The model under review builds one solid part; all positions refer to its coordinate system, in mm. A direction names the side the tool comes from. Give positions to 0.01 mm unless a question says otherwise; leave off trailing zeros. Order: outer loops, then holes, each group sorted by start corner. A loop starts at its lowest first (then second) coordinate and runs counter-clockwise, first axis right, second up. Notation, with made-up numbers: (56, 66.25) - (102, 66.25) arc R20 ccw to (102, 70.25) - close; hole circle Ø2 at (40.5, -0.75). An arc over 180 degrees is marked (long way). Write item = value, one per line. Start each with the question number.
1. For P1, Ø5, axis at y = 38, z = 5.5, coming from the +X side; P2, Ø4.5, axis at x = 55.5, z = 10, coming from the +Y side, all flat-tipped, find the tip position at first contact; note any pin that passes through.
2. Machinability: for faces 1 (the cylindrical face through (126.82, 51.02, 7.4)), 2 (the flat face through (43, 50, 7)), which of the approach directions +Z, -Z, +X, -X, +Y, -Y give a long, thin tool a straight path to every point of the face, cutting with its end or side? Answer none if there is none.
3. We need section A-A, the plane z = 7.5. Give the boundary of the cut face in (x, y).
4. We need section B-B, the plane x = 61.5. Give the boundary of the cut face in (y, z), and give its area (3 significant figures).
5. Wall thickness on probe 1 along Y at (x, z) = (40.5, 5.5); probe 2 along Y at (x, z) = (5.5, 8.5); probe 3 along X at (y, z) = (22.5, 10.5): over which ranges is each line inside the solid? List them lowest first.
6. We need section C-C, the plane y = 17.5. Give the boundary of the cut face in (x, z).
from build123d import *

# Parameters (mm, degrees)
BOSS_EXTRUDE1_DEPTH = 15


with BuildPart() as part:
    # Sketch1 → Boss-Extrude1 (new body)
    with BuildSketch(Plane.XY):
        with BuildLine():
            Line((8, 0), (95.381197846, 0))
            ThreePointArc((95.381197846, 0), (99.381197846, 1.07179677), (102.309401077, 4))
            Line((102.309401077, 4), (126, 45.033320997))
            ThreePointArc((126, 45.033320997), (126.79920338, 51.103873358), (123.07179677, 55.961524227))
            Line((123.07179677, 55.961524227), (97.95706006, 70.461524227))
            ThreePointArc((97.95706006, 70.461524227), (91.886507699, 71.260727607), (87.02885683, 67.533320997))
            Line((87.02885683, 67.533320997), (76.905989232, 50))
            Line((76.905989232, 50), (8, 50))
            ThreePointArc((8, 50), (2.343145751, 47.656854249), (0, 42))
            Line((0, 42), (0, 8))
            ThreePointArc((0, 8), (2.343145751, 2.343145751), (8, 0))
        make_face()
    extrude(amount=BOSS_EXTRUDE1_DEPTH)


solid = part.part
Model answer:
q1.P1 = 123.38
q1.P2 = 50
q2.face_1 = +Z, -Z, +X
q2.face_2 = +Z, -Z, -X, +Y
q3.outline = (0, 8) arc R8 ccw to (8, 0) - (95.38, 0) arc R8 ccw to (102.31, 4) - (126, 45.03) arc R8 ccw to (123.07, 55.96) - (97.96, 70.46) arc R8 ccw to (87.03, 67.53) - (76.91, 50) - (8, 50) arc R8 ccw to (0, 42) - close
q4.outline = (0, 0) - (50, 0) - (50, 15) - (0, 15) - close
q4.area = 750 mm2
q5.probe_1 = 0 to 50
q5.probe_2 = 0.4 to 49.6
q5.probe_3 = 0 to 112.99
q6.outline = (0, 0) - (110.1, 0) - (110.1, 15) - (0, 15) - close
